Could you check a few things on this drawing? It's one solid part, dimensions in mm from its lowest x, y, z. A direction names the side the tool comes from. Round coordinates to 2 decimals unless told otherwise and drop trailing zeros. Loops run counter-clockwise (first coordinate to the right, second up) from the corner with the lowest first, then second, coordinate; pieces in that order, holes last. Notation, with made-up numbers: M -15,3 L 36,3 A27 cw 36,40 Z; hole C 66,-9 d7. An arc over 180 degrees is marked long. Answer as a JSON object with one key per item and string values.
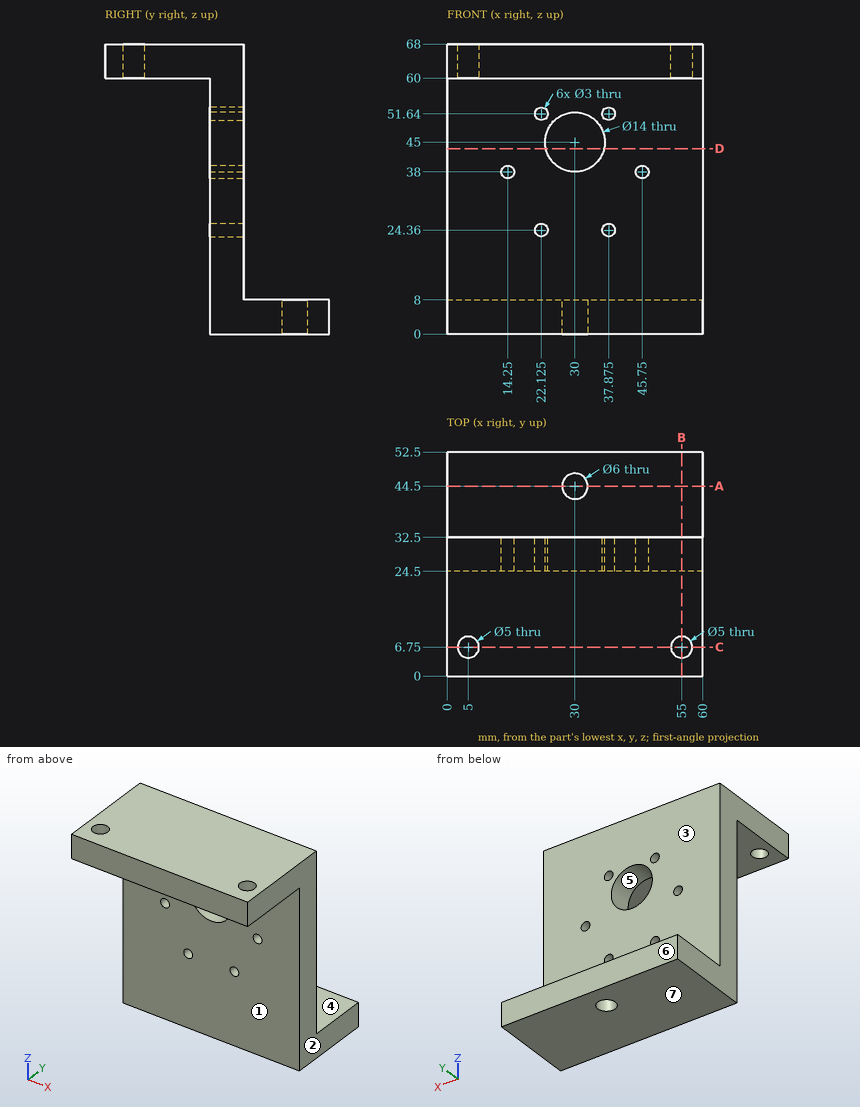
Item 1: I want a section at D-D, the plane z = 43.5. Please give me the cut outline in (x, y).
Resolved:
{"outline": "M 0,24.5 L 23.16,24.5 L 23.16,32.5 L 0,32.5 Z; M 36.84,24.5 L 60,24.5 L 60,32.5 L 36.84,32.5 Z"}
Item 2: I want a section at A-A, the plane y = 44.5. Please give me the cut outline in (x, z).
Resolved:
{"outline": "M 0,0 L 27,0 L 27,8 L 0,8 Z; M 33,0 L 60,0 L 60,8 L 33,8 Z"}
Item 3: I want a section at B-B, the plane x = 55. Please give me the cut outline in (y, z).
Resolved:
{"outline": "M 0,60 L 4.25,60 L 4.25,68 L 0,68 Z; M 9.25,60 L 24.5,60 L 24.5,0 L 52.5,0 L 52.5,8 L 32.5,8 L 32.5,68 L 9.25,68 Z"}
Item 4: Please list where these lines run through material, in increasing order: probe 1 along Z at (x, y) = (14, 27); probe 2 along X at (y, z) = (28, 45); probe 3 along Y at (x, z) = (55, 62.75). Write a range as from..to.
Resolved:
{"probe 1": "0..36.52, 39.48..68", "probe 2": "0..23, 37..60", "probe 3": "0..4.25, 9.25..32.5"}
Item 5: On a 3-axis mill with a long thin cutter (end or side, diameter ignored), from which of +Z, -Z, +X, -X, +Y, -Y can I reach the whole of each face in a straight line? I mean the marked faces 1, 2 and 3. Say none if no direction works.
Resolved:
{"face 1": "-Z, +X, -X, -Y", "face 2": "+Z, -Z, +X, +Y, -Y", "face 3": "+Z, +X, -X, +Y"}
Item 6: I want a section at C-C, the plane y = 6.75. Please give me the cut outline in (x, z), then the cut area to 3 significant figures.
Resolved:
{"outline": "M 0,60 L 2.5,60 L 2.5,68 L 0,68 Z; M 7.5,60 L 52.5,60 L 52.5,68 L 7.5,68 Z; M 57.5,60 L 60,60 L 60,68 L 57.5,68 Z", "area": "400 mm²"}
Item 7: I'm going to push flat-ended pins straight in: pin 1 Ø4 at (y, z) = (29.5, 56.5) entering from -X; pin 2 Ø4 at (x, z) = (14.25, 38) entering from -Y; pin 3 Ø6 at (x, y) = (37, 44) entering from +Z; pin 4 Ø3.5 at (x, z) = (45.75, 38) entering from +Y. Where does each tip first touch, or does it pass through?
Resolved:
{"pin 1": "x = 0", "pin 2": "y = 24.5", "pin 3": "z = 8", "pin 4": "y = 32.5"}
Item 8: If we mould it in two halves opening along Z, with no side actions, what happens to the marked faces 4, 5, 6 and 7? For each: pulls with the +Z half, pulls with the -Z half, needs draft (parallel to the pull), parting line crosses it, or undercut.
Resolved:
{"face 4": "pulls with the +Z half", "face 5": "undercut", "face 6": "needs draft", "face 7": "pulls with the -Z half"}
